from build123d import *

# Parameters (mm, degrees)
F1_DEPTH      = 5
F3_DEPTH      = 1
F3_DEPTH_BACK = 15
F5_DEPTH      = 1
F5_DEPTH_BACK = 59.9


with BuildPart() as f1:
    # F0 (on Right) → F1 (new body, symmetric)
    with BuildSketch(Plane.YZ):
        Polygon((-111.234378, -36.859374), (-41.234378, -36.859374), (-41.234378, 23.140626), align=None)
        Polygon((-41.234378, 23.140626), (-41.234378, -36.859374), (-31.234378, -36.859374), (58.765622, 13.140626), (58.765622, 23.140626), align=None)
    extrude(amount=F1_DEPTH, both=True)

    # F2 (on face) → F3 (join, two sides)
    with BuildSketch(Plane.XY.offset(23.140626)) as f3_sk:
        with BuildLine():
            ThreePointArc((-5, 52.904069), (0, 47.904069), (5, 52.904069))
            ThreePointArc((5, 52.904069), (0, 57.904069), (-5, 52.904069))
        make_face()
    extrude(amount=F3_DEPTH)
    extrude(f3_sk.sketch, amount=-F3_DEPTH_BACK)

    # F4 (on face) → F5 (join, two sides)
    with BuildSketch(Plane.XY.offset(23.140626)) as f5_sk:
        with BuildLine():
            ThreePointArc((0, -41.234378), (3.535534, -39.769912), (5, -36.234378))
            ThreePointArc((5, -36.234378), (0, -31.234378), (-5, -36.234378))
            ThreePointArc((-5, -36.234378), (-3.535534, -39.769912), (0, -41.234378))
        make_face()
    extrude(amount=F5_DEPTH)
    extrude(f5_sk.sketch, amount=-F5_DEPTH_BACK)


solid = f1.part
Can you work these out from the model? Positions are in its coordinate system, mm. A direction names the side the tool comes from. Round coordinates to 2 decimals unless told otherwise and drop trailing zeros. Write each loop counter-clockwise with the first axis right and the second up, starting at its lowest first coordinate (ties: lowest second). Pieces come first, ordered by that corner, then holes. Notation, with made-up numbers: (39.5, 1.5) - (60.5, 1.5) arc R19 cw to (60.5, 7.5) - close; hole circle Ø9 at (20, -29.5). An arc over 180 degrees is marked (long way). Write each question's results on one line, items separated by ' | '. Start each with the question number.
1) Please list where these lines run through material, in increasing order: line 1 (Z direction, x = -2.5, y = 52); line 2 (Y direction, x = 3.25, z = 21.5); line 3 (Z direction, x = 3.25, y = 47).
2) Which directions (+Z, -Z, +X, -X, +Y, -Y) give clear straight access to the entire face, cutting with the end or side of a thin tool? Please do faces 5 (the flat face through (1, 58, 23.141)), 6 (the flat face through (-4, -40, 23.141)), 7 (the flat face through (4, -40, 23.141)).
3) Suppose I cut it at C-C (z = -3). List the corners of the cut face in (x, y) for me.
4) For pin 1 Ø4 at (x, y) = (3.5, 22.5) entering from -Z; pin 2 Ø2 at (x, z) = (-2.5, -29.5) entering from +Y; pin 3 Ø1 at (x, y) = (1.5, -19.5) entering from +Z, each with a flat end and sliding along its axis, tell me the tip position at first contact or that it passes through.
5) We'd pull the mould along Y, two halves only. Please class faces 1 (the cylindrical face through (-0.65, 57.86, 23.63)), 2 (the flat face through (0.1, -75.7, -6.4)), 3 (the flat face through (0, 54, 8.141)), 4 (the flat face through (0, 9, 23.141)): released by +Y, released by -Y, zero draft, split by the parting line, or undercut.
6) Suppose I cut it at B-B (y = -14). List the corners of the cut face in (x, z) for me.
7) Suppose I cut it at A-A (x = 2). List the corners of the cut face in (y, z) for me, and give its area (3 significant figures).
Here are the results:
1) line 1: z = 8.14 to 24.14 | line 2: y = -43.15 to 58.77 | line 3: z = 6.6 to 23.14
2) face 5: +Z, +Y | face 6: +Z, -X, -Y | face 7: +Z, +X, -Y
3) outline: (-5, -71.73) - (5, -71.73) - (5, 29.71) - (-5, 29.71) - close
4) pin 1: stops at z = -8.12 | pin 2: stops at y = -16.19 | pin 3: stops at z = 23.14
5) face 1: undercut | face 2: released by -Y | face 3: zero draft | face 4: undercut
6) outline: (-5, -27.28) - (5, -27.28) - (5, 23.14) - (-5, 23.14) - close
7) outline: (-111.23, -36.86) - (-31.23, -36.86) - (49.77, 8.14) - (57.49, 8.14) - (57.49, 12.43) - (58.77, 13.14) - (58.77, 23.14) - (57.49, 23.14) - (57.49, 24.14) - (48.32, 24.14) - (48.32, 23.14) - (-31.65, 23.14) - (-31.65, 24.14) - (-40.82, 24.14) - (-40.82, 23.14) - (-41.23, 23.14) - close | area: 5,880 mm2
